Solid Edge part; units mm, degrees
sketch "Sketch1" plane through (0, 0, 0) normal (0, 0, 1) x (1, 0, 0)
  line L0 (8.953, 5.2481) -> (3.953, 5.2481)
  line L1 (3.953, 5.2481) -> (3.953, 42.2481)
  line L2 (3.953, 42.2481) -> (71.953, 42.2481)
  line L3 (71.953, 42.2481) -> (71.953, 5.2481)
  line L4 (71.953, 5.2481) -> (66.953, 5.2481)
  line L5 (66.953, 5.2481) -> (66.953, 1.2481)
  line L6 (66.953, 1.2481) -> (52.953, 1.2481)
  line L7 (52.953, 1.2481) -> (52.953, 5.2481)
  line L8 (52.953, 5.2481) -> (44.953, 5.2481)
  line L9 (44.953, 5.2481) -> (44.953, 1.2481)
  line L10 (44.953, 1.2481) -> (30.953, 1.2481)
  line L11 (30.953, 1.2481) -> (30.953, 5.2481)
  line L12 (30.953, 5.2481) -> (22.953, 5.2481)
  line L13 (22.953, 5.2481) -> (22.953, 1.2481)
  line L14 (22.953, 1.2481) -> (8.953, 1.2481)
  line L15 (8.953, 1.2481) -> (8.953, 5.2481)
extrude "Protrusion1" add sketch "Sketch1" along normal blind 4
sketch "Sketch2" plane through (37.953, 21.7481, 4) normal (0, 0, 1) x (1, 0, 0)
  line L0 (-20.5, -10.5) -> (-20.5, -1.5)
  line L1 (-20.5, -1.5) -> (-24, -1.5)
  line L2 (-24, -0.25) -> (-24, -1.5)
  line L3 (-24, -0.25) -> (-24, 1)
  line L4 (-24, 1) -> (-20.5, 1)
  line L5 (-20.5, 1) -> (-20.5, 10)
  line L6 (-20.5, 10) -> (20.5, 10)
  line L7 (20.5, 10) -> (20.5, 1)
  line L8 (20.5, 1) -> (24, 1)
  line L9 (24, 1) -> (24, -1.5)
  line L10 (24, -1.5) -> (20.5, -1.5)
  line L11 (20.5, -1.5) -> (20.5, -10.5)
  line L12 (20.5, -10.5) -> (-20.5, -10.5)
extrude "Recorte_Extrudado_1" cut sketch "Sketch2" against normal blind 11.4351
fillet "Redondo_3" radius 5 2 edges at (71.953, 42.2481, 2) (3.953, 42.2481, 2)
The listing builds one solid part. Answer for the finished solid, in the listing's coordinates (mm). A direction names the side the tool comes from. Round coordinates to 2 decimals unless told otherwise and drop trailing zeros. Order: outer loops, then holes, each group sorted by start corner. A loop starts at its lowest first (then second) coordinate and runs counter-clockwise, first axis right, second up. Notation, with made-up numbers: (-20, 2) -> (37, 2) arc R29 ccw to (37, 35) -> close; hole circle Ø9 at (87.5, -24.5). An arc over 180 degrees is marked (long way). One line per item, written item: value.
Item 1: Find section C-C, the plane y = 21. Give the vertices of the cut face in (x, z).
Taken from the geometry:
outline: (3.95, 0) -> (13.95, 0) -> (13.95, 4) -> (3.95, 4) -> close; (61.95, 0) -> (71.95, 0) -> (71.95, 4) -> (61.95, 4) -> close
Item 2: Given P1, Ø6, axis at x = 52.5, y = 27.5, coming from the +Z side, flat-ended and moving along its own axis, determine where the tip first touches the part or whether it passes through.
Taken from the geometry:
P1: passes through
Item 3: For faces 1 (the flat face through (8.953, 3, 2)), 2 (the flat face through (38, 36, 0)), 3 (the flat face through (58.453, 27, 2)), 4 (the flat face through (27, 5.248, 2)), 5 (the flat face through (66.953, 3, 2)), determine the directions among +Z, -Z, +X, -X, +Y, -Y from which every point of the face is accessible in a straight line to the end or side of a thin tool.
Taken from the geometry:
face 1: +Z, -Z, -X, -Y
face 2: -Z, +X, -X, +Y, -Y
face 3: +Z, -Z
face 4: +Z, -Z, -Y
face 5: +Z, -Z, +X, -Y
Item 4: For a pull along Y with two mould halves and no side action, classify faces 6 (the cylindrical face through (70.53, 40.74, 2.03)), 7 (the flat face through (6, 5.248, 2)), 8 (the flat face through (60, 20.248, 2)) as released by +Y, released by -Y, zero draft, split by the parting line, or undercut.
Taken from the geometry:
face 6: released by +Y
face 7: released by -Y
face 8: undercut
Item 5: Straight lines are drawn through the part: L1, parallel to X at y = 31, z = 1.7; L2, parallel to Y at x = 47, z = 1.3; L3, parallel to Y at x = 21.5, z = 0.6. For each, find the intervals that lie inside material, in ascending order.
Taken from the geometry:
L1: x = 3.95 to 17.45, 58.45 to 71.95
L2: y = 5.25 to 11.25, 31.75 to 42.25
L3: y = 1.25 to 11.25, 31.75 to 42.25
Item 6: Find section A-A, the plane x = 61. Give the vertices of the cut face in (y, z).
Taken from the geometry:
outline: (1.25, 0) -> (20.25, 0) -> (20.25, 4) -> (1.25, 4) -> close; (22.75, 0) -> (42.25, 0) -> (42.25, 4) -> (22.75, 4) -> close
